Verification items for the finished model (mm, model axes). A direction names the side the tool comes from. Give positions to 0.01 mm unless a question says otherwise; leave off trailing zeros. Order: outer loops, then holes, each group sorted by start corner. A loop starts at its lowest first (then second) coordinate and runs counter-clockwise, first axis right, second up.
from build123d import *

# Parameters (mm, degrees)
BOSS_EXTRUDE1_DEPTH = 2.9972
SKETCH2_R           = 3
BOSS_EXTRUDE2_DEPTH = 11.176
SKETCH3_R           = 4.4958
BOSS_EXTRUDE3_DEPTH = 1.016
CUT_EXTRUDE1_DEPTH  = 1.524
SKETCH5_R           = 3.556
CUT_EXTRUDE2_DEPTH  = 1.9812
SKETCH6_R           = 1.1176
CUT_EXTRUDE3_DEPTH  = 32.262860272
SKETCH9_R           = 0.9906
CUT_EXTRUDE4_DEPTH  = 10.16
SCALE1_SCALE        = 0.6


with BuildPart() as part:
    # Sketch1 → Boss-Extrude1 (new body)
    with BuildSketch(Plane(origin=(0, 0, 0), x_dir=(0, 0, -1), z_dir=(1, 0, 0))):
        with BuildLine():
            Line((24.769539012, 3.626266444), (5.771274976, 5.288399174))
            ThreePointArc((5.771274976, 5.288399174), (0, 0), (5.771274976, -5.288399174))
            Line((5.771274976, -5.288399174), (24.769539012, -3.626266444))
            ThreePointArc((24.769539012, -3.626266444), (28.0924, 0), (24.769539012, 3.626266444))
        make_face()
    extrude(amount=BOSS_EXTRUDE1_DEPTH)

    # Sketch2 → Boss-Extrude2 (add)
    with BuildSketch(Plane.ZY):
        with Locations(Location((-5.3086, 0, 0), (0, 0, 180))):
            Circle(SKETCH2_R)
    extrude(amount=BOSS_EXTRUDE2_DEPTH)

    # Sketch3 → Boss-Extrude3 (add)
    with BuildSketch(Plane.ZY):
        with Locations(Location((-5.3086, 0, 0), (0, 0, 180))):
            Circle(SKETCH3_R)
    extrude(amount=BOSS_EXTRUDE3_DEPTH)

    # Sketch4 → Cut-Extrude1 (cut)
    with BuildSketch(Plane(origin=(2.9972, 0, 0), x_dir=(0, 0, -1), z_dir=(1, 0, 0))):
        with BuildLine():
            Line((24.703126336, 2.867166085), (5.7048623, 4.529298814))
            ThreePointArc((5.7048623, 4.529298814), (0.762, 0), (5.7048623, -4.529298814))
            Line((5.7048623, -4.529298814), (24.703126336, -2.867166085))
            ThreePointArc((24.703126336, -2.867166085), (27.3304, 0), (24.703126336, 2.867166085))
        make_face()
    extrude(amount=-CUT_EXTRUDE1_DEPTH, mode=Mode.SUBTRACT)

    # Sketch5 → Cut-Extrude2 (cut)
    with BuildSketch(Plane(origin=(1.4732, 0, 0), x_dir=(0, 0, -1), z_dir=(1, 0, 0))):
        with Locations((5.3086, 0)):
            Circle(SKETCH5_R)
    extrude(amount=-CUT_EXTRUDE2_DEPTH, mode=Mode.SUBTRACT)

    # Sketch6 → Cut-Extrude3 (cut, through all)
    with BuildSketch(Plane(origin=(1.4732, 0, 0), x_dir=(0, 0, -1), z_dir=(1, 0, 0))):
        with Locations((21.2344, 0)):
            Circle(SKETCH6_R)
    extrude(amount=-CUT_EXTRUDE3_DEPTH, mode=Mode.SUBTRACT)

    # Sketch9 → Cut-Extrude4 (cut)
    with BuildSketch(Plane(origin=(0, 4.943430386, -8.562272593), x_dir=(-1, 0, 0), z_dir=(0, 0.5000000000000044, -0.866025403784436))):
        with Locations(Location((6.134133556, -3.622041732, 0), (0, 0, 90))):
            Circle(SKETCH9_R)
    extrude(amount=-CUT_EXTRUDE4_DEPTH, mode=Mode.SUBTRACT)


with BuildPart() as part_1:
    # Scale1: scaled about (-1.924771694, 0.020710346, -10.183561465)
    add(part.part.scale(SCALE1_SCALE).moved(Location((-0.769908678, 0.008284138, -4.073424586))))


solid = part_1.part
(1) Go/stop test with flat-tipped pins: pin 1 (1.5 mm diameter, centred on y = 0.01, z = -16.81, fed in from -X); pin 2 (3 mm diameter, centred on x = -6.5, y = -2, fed in from +Z); pin 3 (3.5 mm diameter, centred on y = 0, z = -8, fed in from +X). Record where each tip stops, or that it passes through.
Solved:
pin 1: stops at x = -0.77
pin 2: stops at z = -5.53
pin 3: stops at x = 0.11
(2) Section check A-A, the plane x = 0.5. Enter the section's corners in (y, z), then the cut area to 3 significant figures.
Solved:
outline: (-3.16, -7.54) - (-2.17, -18.94) arc R2.18 ccw to (2.18, -18.94) - (3.18, -7.54) arc R3.19 ccw (long way) to start; hole (-2.71, -7.5) - (-1.71, -18.9) arc R1.73 ccw to (1.73, -18.9) - (2.73, -7.5) arc R2.73 ccw (long way) to start
area: 17.6 mm2
(3) Release check for a two-part mould opening along Z. For faces 4 (the flat face through (-0.77, 0, -14)), 5 (the flat face through (0.58, 2.22, -13.28)), 6 (the cylindrical face through (0.12, -0.04, -20.93)) record: pulls with the +Z half, pulls with the -Z half, needs draft (parallel to the pull), parting line crosses it, or undercut.
Solved:
face 4: needs draft
face 5: undercut
face 6: pulls with the -Z half
(4) Section check C-C, the plane y = 2.5. Enter the section's corners in (x, z).
Solved:
outline: (-1.38, -8.29) - (-0.77, -8.29) - (-0.77, -15.32) - (1.03, -15.32) - (1.03, -10.08) - (0.11, -10.08) - (0.11, -6.15) - (1.03, -6.15) - (1.03, -5.27) - (-0.77, -5.27) - (-0.77, -6.23) - (-1.38, -6.23) - close
(5) Section check D-D, the plane z = -11.25. Enter the section's corners in (x, y), then the cut area to 3 significant figures.
Solved:
outline: (-0.77, -2.84) - (1.03, -2.84) - (1.03, -2.38) - (0.11, -2.38) - (0.11, 2.4) - (1.03, 2.4) - (1.03, 2.86) - (-0.77, 2.86) - close
area: 5.87 mm2
(6) Section check B-B, the plane z = -17. Enter the section's corners in (x, y).
Solved:
outline: (-0.77, -2.34) - (1.03, -2.34) - (1.03, -1.88) - (0.11, -1.88) - (0.11, -0.64) - (-0.77, -0.64) - close; (-0.77, 0.65) - (0.11, 0.65) - (0.11, 1.89) - (1.03, 1.89) - (1.03, 2.35) - (-0.77, 2.35) - close
(7) Scan lines: line 1 (Z direction, x = 0, y = 0) (3 decimals); line 2 (X direction, y = -3, z = -8.5); line 3 (X direction, y = 1, z = -5.5). Record each from-to range of solid material in increasing order.
Solved:
line 1: z = -20.929 to -17.485, -16.144 to -9.392, -5.125 to -4.073
line 2: x = -0.77 to 1.03
line 3: x = -1.38 to -1.07
(8) Set-up check for faces 1 (the flat face through (1.028, -2.57, -12.46)), 2 (the cylindrical face through (-4.385, 1.765, -6.868)), 3 (the flat face through (0.578, -2.218, -13.116)): record each of +Z, -Z, +X, -X, +Y, -Y from which the full face is reachable in a straight line by a thin tool's end or side.
Solved:
face 1: +Z, -Z, +X, +Y, -Y
face 2: -X
face 3: +X
